Can you work these out from the drawing? Everything is in mm from the part's minimum corner. Give positions to 0.01 mm unless a question says otherwise; leave off trailing zeros. Order: outer loops, then holes, each group sorted by start corner. A loop starts at its lowest first (then second) coordinate and runs counter-clockwise, first axis right, second up. Notation, with made-up numbers: (38.5, -19.5) - (71.5, -19.5) arc R22 ccw to (71.5, 12.5) - close; hole circle Ø3 at (84, 19). An arc over 180 degrees is marked (long way). One line per question, with ' | ' between items.
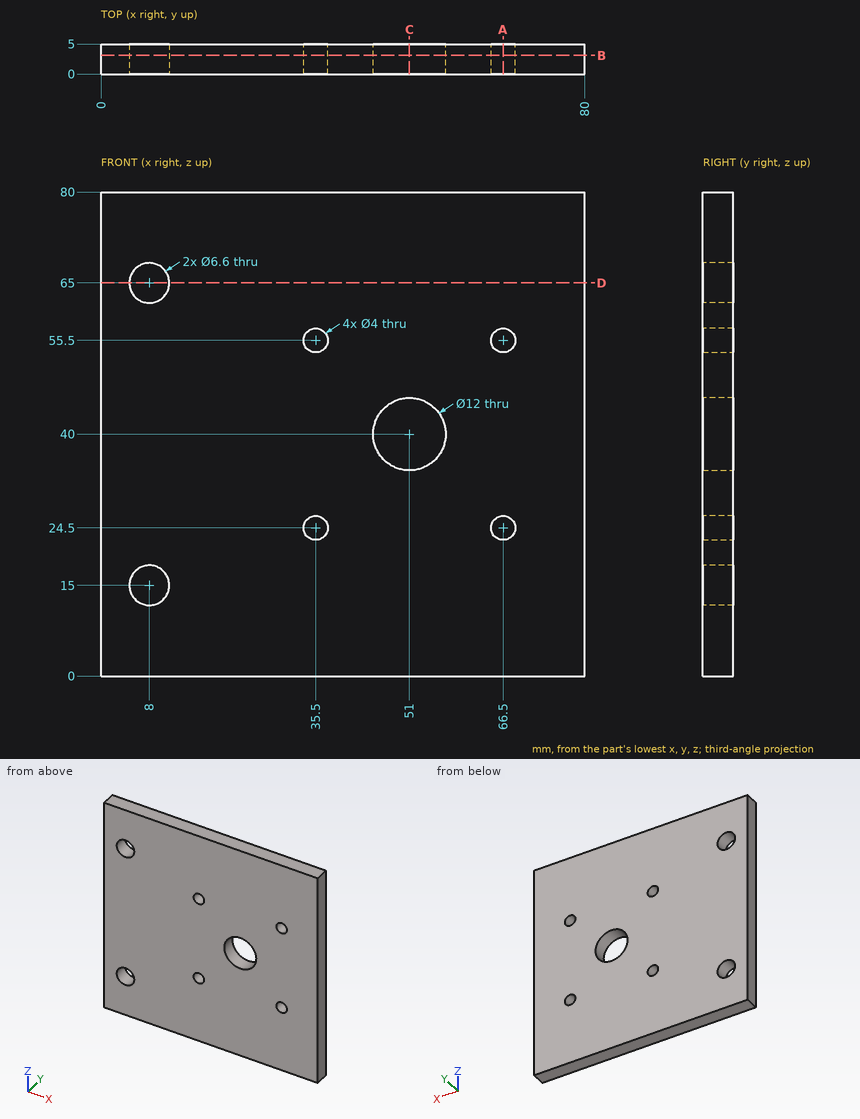
(1) Imagine slicing it at D-D (z = 65). List the corners of the cut face in (x, y) for me.
Answer below:
outline: (0, 0) - (4.7, 0) - (4.7, 5) - (0, 5) - close; (11.3, 0) - (80, 0) - (80, 5) - (11.3, 5) - close
(2) If I drill on line 1 (Z direction, x = 8, y = 3.2); line 2 (X direction, y = 2.3, z = 15); line 3 (X direction, y = 2.35, z = 24.5), over which ranges is the centre line in solid material (lowest first)?
Answer below:
line 1: 0 to 11.7, 18.3 to 61.7, 68.3 to 80 | line 2: 0 to 4.7, 11.3 to 80 | line 3: 0 to 33.5, 37.5 to 64.5, 68.5 to 80
(3) Imagine slicing it at A-A (x = 66.5). List the corners of the cut face in (y, z) for me.
Answer below:
outline: (0, 0) - (5, 0) - (5, 22.5) - (0, 22.5) - close; (0, 26.5) - (5, 26.5) - (5, 53.5) - (0, 53.5) - close; (0, 57.5) - (5, 57.5) - (5, 80) - (0, 80) - close
(4) Imagine slicing it at B-B (y = 3.1). List the corners of the cut face in (x, z) for me, and give its area (3 significant figures).
Answer below:
outline: (0, 0) - (80, 0) - (80, 80) - (0, 80) - close; hole circle Ø6.6 at (8, 15); hole circle Ø6.6 at (8, 65); hole circle Ø4 at (35.5, 24.5); hole circle Ø4 at (35.5, 55.5); hole circle Ø12 at (51, 40); hole circle Ø4 at (66.5, 24.5); hole circle Ø4 at (66.5, 55.5) | area: 6,170 mm^2
(5) Imagine slicing it at C-C (x = 51). List the corners of the cut face in (y, z) for me, and give its area (3 significant figures).
Answer below:
outline: (0, 0) - (5, 0) - (5, 34) - (0, 34) - close; (0, 46) - (5, 46) - (5, 80) - (0, 80) - close | area: 340 mm^2
